from build123d import *

# Parameters (mm, degrees)
F0_W     = 12.7
F0_H     = 25.4
F1_DEPTH = 25.4
F2_DEPTH = 25.4
F3_W     = 12.7
F3_H     = 6.35
F4_DEPTH = 25.4


with BuildPart() as f1:
    # F0 (on Front) → F1 (new body)
    with BuildSketch(Plane.XZ):
        Polygon((-37.512038, 12.7), (-37.512038, 0), (25.987962, 0), (25.987962, 12.7), (-24.812038, 12.7), align=None)
        with Locations((-31.162038, 25.4)):
            Rectangle(F0_W, F0_H)
    extrude(amount=F1_DEPTH)

    # F0 (on Front) → F2 (join)
    with BuildSketch(Plane.XZ):
        Polygon((-37.512038, 12.7), (-37.512038, 0), (25.987962, 0), (25.987962, 12.7), (-24.812038, 12.7), align=None)
        with Locations((-31.162038, 25.4)):
            Rectangle(F0_W, F0_H)
    extrude(amount=F2_DEPTH)

    # F3 (on face) → F4 (cut)
    with BuildSketch(Plane.YZ.offset(-24.812038)):
        with BuildLine():
            ThreePointArc((-19.05, 31.75), (-12.7, 25.4), (-6.35, 31.75))
            Line((-6.35, 31.75), (-19.05, 31.75))
        make_face()
        with Locations((-12.7, 34.925)):
            Rectangle(F3_W, F3_H)
    extrude(amount=-F4_DEPTH, mode=Mode.SUBTRACT)


solid = f1.part
The listing builds one solid part. Answer for the finished solid, in the listing's coordinates (mm). A direction names the side the tool comes from. Coordinates: 2 decimals unless noted, no trailing zeros. Loops run counter-clockwise (first coordinate to the right, second up) from the corner with the lowest first, then second, coordinate; pieces in that order, holes last. Notation, with made-up numbers: (35, 18.5) -> (57, 18.5) arc R18 cw to (57, 40.5) -> close; hole circle Ø7 at (54.25, 42). An arc over 180 degrees is marked (long way). Answer in a Markdown table with one row per item. Add a question column.
1. For faces 1 (the flat face through (-6, -13, 0)), 2 (the flat face through (-31, -19.05, 35)), 3 (the flat face through (1, -13, 12.7)), determine the directions among +Z, -Z, +X, -X, +Y, -Y from which every point of the face is accessible in a straight line to the end or side of a thin tool.
2. The part is cut by section B-B, the plane z = 16. Write down the section's boundary in (x, y).
3. The part is cut by section A-A, the plane y = -4.25. Write down the section's boundary in (x, z), then the cut area to 3 significant figures.
4. The part is cut by section D-D, the plane y = -12.7. Write down the section's boundary in (x, z), then the cut area to 3 significant figures.
5. The part is cut by section C-C, the plane x = -12. Write down the section's boundary in (y, z), then the cut area to 3 significant figures.
6. Consider line 1 (Z direction, x = 22, y = -21); line 2 (X direction, y = -4.5, z = 20.5). Determine where each line is inside the solid, lowest interval first. Write a range as [from, to].
7. Flat-ended cylindrical pins translate along their axes: P1, Ø3, axis at x = -19, y = -22.5, coming from the +Z side; P2, Ø12.5, axis at y = -10, z = 23, coming from the +X side. Find the tip coordinate at first contact, or state that the pin passes through.
Answer below:
| question | item | result |
|---|---|---|
| 1 | face 1 | -Z, +X, -X, +Y, -Y |
| 1 | face 2 | +Z, +X, -X |
| 1 | face 3 | +Z, +X, +Y, -Y |
| 2 | outline | (-37.51, -25.4) -> (-24.81, -25.4) -> (-24.81, 0) -> (-37.51, 0) -> close |
| 3 | outline | (-37.51, 0) -> (25.99, 0) -> (25.99, 12.7) -> (-24.81, 12.7) -> (-24.81, 38.1) -> (-37.51, 38.1) -> close |
| 3 | area | 1,130 mm2 |
| 4 | outline | (-37.51, 0) -> (25.99, 0) -> (25.99, 12.7) -> (-24.81, 12.7) -> (-24.81, 25.4) -> (-37.51, 25.4) -> close |
| 4 | area | 968 mm2 |
| 5 | outline | (-25.4, 0) -> (0, 0) -> (0, 12.7) -> (-25.4, 12.7) -> close |
| 5 | area | 323 mm2 |
| 6 | line 1 | [0, 12.7] |
| 6 | line 2 | [-37.51, -24.81] |
| 7 | P1 | z = 12.7 |
| 7 | P2 | x = -24.81 |
